Can you work these out from the model? Positions are in its coordinate system, mm. Face numbers are marked on the shaded views. A direction names the side the tool comes from. Give positions to 0.01 mm unless a question says otherwise; leave off trailing zeros. Order: outer loops, then holes, each group sorted by start corner. A loop starts at its lowest first (then second) coordinate and runs counter-clockwise, first axis right, second up. Notation, with made-up numbers: M 85.25,21.25 L 89.25,21.25 A15 ccw 89.25,39.25 Z; hole C -0.5,12.5 d11. An arc over 180 degrees is marked long. Answer as a JSON object with one key per item and string values.
```python
from build123d import *

# Parameters (mm, degrees)
SKETCH1_W                 = 29
SKETCH1_H                 = 29
BOSS_EXTRUDE1_DEPTH       = 30
M2X0_4_TAPPED_HOLE1_D     = 1.6
M2X0_4_TAPPED_HOLE1_DEPTH = 2.5
M2X0_4_TAPPED_HOLE1_TIP   = 0.480688495
M3X0_5_TAPPED_HOLE1_D     = 2.5
M3X0_5_TAPPED_HOLE1_DEPTH = 2.8
M3X0_5_TAPPED_HOLE1_TIP   = 0.751075774
M3X0_5_TAPPED_HOLE2_D     = 2.5
M3X0_5_TAPPED_HOLE2_DEPTH = 2.5
M3X0_5_TAPPED_HOLE2_TIP   = 0.751075774
M2X0_4_TAPPED_HOLE2_D     = 1.6
M2X0_4_TAPPED_HOLE2_DEPTH = 2.5
M2X0_4_TAPPED_HOLE2_TIP   = 0.480688495
M2X0_4_TAPPED_HOLE3_D     = 1.6
M2X0_4_TAPPED_HOLE3_DEPTH = 2
M2X0_4_TAPPED_HOLE3_TIP   = 0.480688495
SKETCH12_R                = 1.000276531
SKETCH12_R_2              = 1
SKETCH12_W                = 10
SKETCH12_H                = 2
CUT_EXTRUDE4_DEPTH        = 3
SKETCH13_R                = 4.5
BOSS_EXTRUDE2_DEPTH       = 4
SKETCH14_R                = 14.5
SKETCH14_R_2              = 13.5
BOSS_EXTRUDE3_DEPTH       = 4


with BuildPart() as part:
    # Sketch1 → Boss-Extrude1 (new body)
    with BuildSketch(Plane.XY):
        Rectangle(SKETCH1_W, SKETCH1_H)
    extrude(amount=BOSS_EXTRUDE1_DEPTH)

    # M2x0.4 Tapped Hole1
    with Locations(Plane(origin=(0, 14.5, 0), x_dir=(1, 0, 0), z_dir=(0, 1, 0))):
        with Locations((-6, -28), (6, -28)):
            Hole(M2X0_4_TAPPED_HOLE1_D / 2, depth=M2X0_4_TAPPED_HOLE1_DEPTH)
            with Locations((0, 0, -(M2X0_4_TAPPED_HOLE1_DEPTH + M2X0_4_TAPPED_HOLE1_TIP / 2))):  # 118° drill point
                Cone(0, M2X0_4_TAPPED_HOLE1_D / 2, M2X0_4_TAPPED_HOLE1_TIP, mode=Mode.SUBTRACT)

    # M3x0.5 Tapped Hole1
    with Locations(Plane(origin=(0, -14.5, 0), x_dir=(-1, 0, 0), z_dir=(0, -1, 0))):
        with Locations((-10, -27), (10, -27)):
            Hole(M3X0_5_TAPPED_HOLE1_D / 2, depth=M3X0_5_TAPPED_HOLE1_DEPTH)
            with Locations((0, 0, -(M3X0_5_TAPPED_HOLE1_DEPTH + M3X0_5_TAPPED_HOLE1_TIP / 2))):  # 118° drill point
                Cone(0, M3X0_5_TAPPED_HOLE1_D / 2, M3X0_5_TAPPED_HOLE1_TIP, mode=Mode.SUBTRACT)

    # M3x0.5 Tapped Hole2
    with Locations(Plane(origin=(0, -14.5, 0), x_dir=(-1, 0, 0), z_dir=(0, -1, 0))):
        with Locations((0, -3.3)):
            Hole(M3X0_5_TAPPED_HOLE2_D / 2, depth=M3X0_5_TAPPED_HOLE2_DEPTH)
            with Locations((0, 0, -(M3X0_5_TAPPED_HOLE2_DEPTH + M3X0_5_TAPPED_HOLE2_TIP / 2))):  # 118° drill point
                Cone(0, M3X0_5_TAPPED_HOLE2_D / 2, M3X0_5_TAPPED_HOLE2_TIP, mode=Mode.SUBTRACT)

    # M2x0.4 Tapped Hole2
    with Locations(Plane(origin=(0, -14.5, 0), x_dir=(-1, 0, 0), z_dir=(0, -1, 0))):
        with Locations((-6, -25.5), (6, -25.5)):
            Hole(M2X0_4_TAPPED_HOLE2_D / 2, depth=M2X0_4_TAPPED_HOLE2_DEPTH)
            with Locations((0, 0, -(M2X0_4_TAPPED_HOLE2_DEPTH + M2X0_4_TAPPED_HOLE2_TIP / 2))):  # 118° drill point
                Cone(0, M2X0_4_TAPPED_HOLE2_D / 2, M2X0_4_TAPPED_HOLE2_TIP, mode=Mode.SUBTRACT)

    # M2x0.4 Tapped Hole3
    with Locations(Plane(origin=(0, -14.5, 0), x_dir=(-1, 0, 0), z_dir=(0, -1, 0))):
        with Locations((-6, -3.3), (6, -3.3)):
            Hole(M2X0_4_TAPPED_HOLE3_D / 2, depth=M2X0_4_TAPPED_HOLE3_DEPTH)
            with Locations((0, 0, -(M2X0_4_TAPPED_HOLE3_DEPTH + M2X0_4_TAPPED_HOLE3_TIP / 2))):  # 118° drill point
                Cone(0, M2X0_4_TAPPED_HOLE3_D / 2, M2X0_4_TAPPED_HOLE3_TIP, mode=Mode.SUBTRACT)

    # Sketch12 → Cut-Extrude4 (cut)
    with BuildSketch(Plane(origin=(0, 0, 0), x_dir=(-1, 0, 0), z_dir=(0, 0, -1))):
        with Locations((6.5, -10.000276531)):
            Circle(SKETCH12_R)
        with Locations((-6.5, -10)):
            Circle(SKETCH12_R_2)
        with Locations((0, -10)):
            Rectangle(SKETCH12_W, SKETCH12_H)
    extrude(amount=-CUT_EXTRUDE4_DEPTH, mode=Mode.SUBTRACT)

    # Sketch13 → Boss-Extrude2 (add)
    with BuildSketch(Plane(origin=(0, 0, 0), x_dir=(-1, 0, 0), z_dir=(0, 0, -1))):
        with Locations((-8.5, 8.5)):
            Circle(SKETCH13_R)
    extrude(amount=BOSS_EXTRUDE2_DEPTH)

    # Sketch14 → Boss-Extrude3 (add)
    with BuildSketch(Plane.XY.offset(30)):
        Circle(SKETCH14_R)
        Circle(SKETCH14_R_2, mode=Mode.SUBTRACT)
    extrude(amount=BOSS_EXTRUDE3_DEPTH)


solid = part.part
```
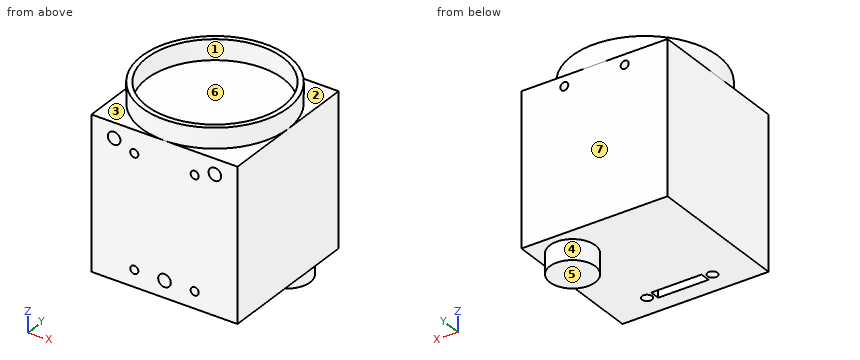
1) I need wall thicknesses on L1, parallel to X at y = -12.8, z = 27; L2, parallel to X at y = 13.5, z = 28; L3, parallel to Z at x = -6, y = -12.75. Which ranges of each line are inside material? Lowest first, please.
Results found:
{"L1": "x = -14.5 to -11.25, -8.75 to 8.75, 11.25 to 14.5", "L2": "x = -14.5 to -6.8, -5.2 to 5.2, 6.8 to 14.5", "L3": "z = 0 to 2.5, 4.1 to 24.7, 26.3 to 34"}
2) I'm going to push flat-ended pins straight in: pin 1 Ø2 at (x, y) = (-4, 5) entering from +Z; pin 2 Ø1 at (x, y) = (-7, -9.5) entering from -Z; pin 3 Ø1.3 at (x, z) = (6, 28) entering from +Y. Where does each tip first touch, or does it pass through?
Results found:
{"pin 1": "stops at z = 30", "pin 2": "stops at z = 0", "pin 3": "stops at y = 11.91"}
3) I want a section at B-B on y = -6.5. Write out the boundary of the cut face in (x, z).
Results found:
{"outline": "M -14.5,0 L 14.5,0 L 14.5,30 L 12.96,30 L 12.96,34 L 11.83,34 L 11.83,30 L -11.83,30 L -11.83,34 L -12.96,34 L -12.96,30 L -14.5,30 Z"}
4) Thinking about a two-plate mould opening in Y: for the marked faces 5, 6 and 7, which applies, pulls with the +Y half, pulls with the -Y half, needs draft (parallel to the pull), parting line crosses it, or undercut?
Results found:
{"face 5": "needs draft", "face 6": "undercut", "face 7": "pulls with the +Y half"}
5) I want a section at D-D on y = 5.5. Write out the boundary of the cut face in (x, z), and give its area (3 significant figures).
Results found:
{"outline": "M -14.5,0 L 5.15,0 L 5.15,-4 L 11.85,-4 L 11.85,0 L 14.5,0 L 14.5,30 L 13.42,30 L 13.42,34 L 12.33,34 L 12.33,30 L -12.33,30 L -12.33,34 L -13.42,34 L -13.42,30 L -14.5,30 Z", "area": "906 mm²"}
6) For the marked faces 1, 2, 3 and 4, which set-ups out of +Z, -Z, +X, -X, +Y, -Y let a thin tool reach every point of the face, with its end or its side?
Results found:
{"face 1": "+Z", "face 2": "+Z, +X, +Y", "face 3": "+Z, -X, -Y", "face 4": "-Z"}
7) I want a section at C-C on y = 8.5. Write out the boundary of the cut face in (x, z).
Results found:
{"outline": "M -14.5,0 L 4,0 L 4,-4 L 13,-4 L 13,0 L 14.5,0 L 14.5,30 L 11.75,30 L 11.75,34 L 10.49,34 L 10.49,30 L -10.49,30 L -10.49,34 L -11.75,34 L -11.75,30 L -14.5,30 Z"}
8) I want a section at A-A on z = 30.5. Write out the boundary of the cut face in (x, y).
Results found:
{"outline": "C 0,0 d29; hole C 0,0 d27"}
